Read the model definition and answer for the solid it produces. Units are mm, in the model's axes. A direction names the side the tool comes from. Coordinates: 2 decimals unless noted, no trailing zeros. Write each loop counter-clockwise with the first axis right and the second up, starting at its lowest first coordinate (ties: lowest second). Pieces come first, ordered by that corner, then holes. Notation, with made-up numbers: (0, -24) - (59, -24) arc R33 cw to (59, 11) - close; hole circle Ø2 at (-25.5, -36.5). An arc over 180 degrees is marked (long way). Return JSON: item names as keys, results as strings.
```python
from build123d import *
from OCP.BRepFilletAPI import BRepFilletAPI_MakeChamfer

# Parameters (mm, degrees)
SKETCH1_R           = 4
SKETCH1_R_2         = 1.6
BOSS_EXTRUDE1_DEPTH = 23
SKETCH3_W           = 13.555932204
SKETCH3_H           = 6
SKETCH3_R           = 1.6
CUT_EXTRUDE1_DEPTH  = 2
BOSS_EXTRUDE2_DEPTH = 4
CHAMFER1_SIZE       = 1.5
CHAMFER1_SIZE_2     = 1.062746067


with BuildPart() as part:
    # Sketch1 → Boss-Extrude1 (new body)
    with BuildSketch(Plane(origin=(0, 0, 0), x_dir=(1, 0, 0), z_dir=(0, 1, 0))):
        with Locations(Location((0, 0, 0), (0, 0, 270))):
            Circle(SKETCH1_R)
        with Locations(Location((0, 0, 0), (0, 0, 270))):
            Circle(SKETCH1_R_2, mode=Mode.SUBTRACT)
    extrude(amount=BOSS_EXTRUDE1_DEPTH)

    # Sketch3 → Cut-Extrude1 (cut)
    with BuildSketch(Plane.XZ):
        Rectangle(SKETCH3_W, SKETCH3_H)
        with Locations(Location((0, 0, 0), (0, 0, 270))):
            Circle(SKETCH3_R, mode=Mode.SUBTRACT)
    extrude(amount=-CUT_EXTRUDE1_DEPTH, mode=Mode.SUBTRACT)

    # Sketch5 → Boss-Extrude2 (add)
    with BuildSketch(Plane.XZ):
        with BuildLine():
            Line((-4.609772229, 3), (4.609772229, 3))
            ThreePointArc((4.609772229, 3), (0, 5.5), (-4.609772229, 3))
        make_face()
        with BuildLine():
            Line((4.609772229, -3), (-4.609772229, -3))
            ThreePointArc((-4.609772229, -3), (0, -5.5), (4.609772229, -3))
        make_face()
    extrude(amount=-BOSS_EXTRUDE2_DEPTH)

    # Chamfer1
    chamfer1_edges_1 = [part.edges().sort_by_distance(p)[0] for p in [
        (2.645751311, 3, -3),
    ]]
    chamfer1_side_1 = [part.faces().sort_by_distance(p)[0] for p in [
        (2.667006232, 3, -3),
    ]]
    chamfer1_edges_2 = [part.edges().sort_by_distance(p)[0] for p in [
        (-2.645751311, 3, -3),
    ]]
    chamfer1_side_2 = [part.faces().sort_by_distance(p)[0] for p in [
        (-2.667006232, 3, -3),
    ]]
    chamfer1_edges_3 = [part.edges().sort_by_distance(p)[0] for p in [
        (2.645751311, 3, 3),
    ]]
    chamfer1_side_3 = [part.faces().sort_by_distance(p)[0] for p in [
        (2.667006232, 3, 3),
    ]]
    chamfer1_edges_4 = [part.edges().sort_by_distance(p)[0] for p in [
        (-2.645751311, 3, 3),
    ]]
    chamfer1_side_4 = [part.faces().sort_by_distance(p)[0] for p in [
        (-2.667006232, 3, 3),
    ]]
    chamfer1_edges_5 = [part.edges().sort_by_distance(p)[0] for p in [
        (1.414213562, 4, 3.741657387),
        (0, 4, -4),
    ]]
    chamfer1 = BRepFilletAPI_MakeChamfer(part.part.solid().wrapped)
    for e in chamfer1_edges_1:
        chamfer1.Add(CHAMFER1_SIZE - 0.0001, CHAMFER1_SIZE_2 - 0.0001, e.wrapped, chamfer1_side_1[0].wrapped)
    for e in chamfer1_edges_2:
        chamfer1.Add(CHAMFER1_SIZE - 0.0001, CHAMFER1_SIZE_2 - 0.0001, e.wrapped, chamfer1_side_2[0].wrapped)
    for e in chamfer1_edges_3:
        chamfer1.Add(CHAMFER1_SIZE - 0.0001, CHAMFER1_SIZE_2 - 0.0001, e.wrapped, chamfer1_side_3[0].wrapped)
    for e in chamfer1_edges_4:
        chamfer1.Add(CHAMFER1_SIZE - 0.0001, CHAMFER1_SIZE_2 - 0.0001, e.wrapped, chamfer1_side_4[0].wrapped)
    for e in chamfer1_edges_5:
        chamfer1.Add(CHAMFER1_SIZE - 0.0001, e.wrapped)
    add(Compound.cast(chamfer1.Shape()), mode=Mode.REPLACE)  # a hair under: the kernel refuses the full size


solid = part.part
```
(1) A cutting plane is placed at A-A (y = 3). Determine the outline of the cut face in (x, z), and give its area (3 significant figures).
Answer:
{"outline": "(-4.61, -3) arc R5.5 ccw to (4.61, -3) - (4.15, -3) - (3.34, -2.2) arc R4 ccw to (3.34, 2.2) - (4.15, 3) - (4.61, 3) arc R5.5 ccw to (-4.61, 3) - (-4.15, 3) - (-3.34, 2.2) arc R4 ccw to (-3.34, -2.2) - (-4.15, -3) - close; hole circle Ø3.2 at (0, 0)", "area": "69.7 mm²"}
(2) Flat-ended cylindrical pins translate along their axes: P1, Ø4, axis at y = 10, z = -3.5, coming from the +X side; P2, Ø6, axis at y = 16.5, z = -2, coming from the -X side; P3, Ø1.5, axis at y = 2.5, z = 0.5, coming from the +X side. Find the tip coordinate at first contact, or state that the pin passes through.
Answer:
{"P1": "x = 3.71", "P2": "x = -4", "P3": "x = 4"}
(3) Straight lines are drawn through the part: line 1 (X direction, y = 6.75, z = 0); line 2 (Y direction, x = 2.25, z = 1.5); line 3 (X direction, y = 3.75, z = -1.25). For each, find the intervals that lie inside material, in ascending order. Write a range as from..to.
Answer:
{"line 1": "-4..-1.6, 1.6..4", "line 2": "2..23", "line 3": "-3.8..-1, 1..3.8"}
(4) Determine the mould class of faces 1 (the face through (-2, 2, 0)), 2 (the face through (0, 0, -4)), 3 (the face through (0.1, 5.1, 4.4)) for opening direction Z: +Z half, -Z half, draft (parallel to the pull), parting line (faces both ways), or undercut.
Answer:
{"face 1": "undercut", "face 2": "draft", "face 3": "+Z half"}
(5) A cutting plane is placed at B-B (z = 0). Determine the outline of the cut face in (x, y), and give its area (3 significant figures).
Answer:
{"outline": "(-4, 2) - (-1.6, 2) - (-1.6, 23) - (-4, 23) - close; (1.6, 2) - (4, 2) - (4, 23) - (1.6, 23) - close", "area": "101 mm²"}
(6) A cutting plane is placed at C-C (y = 5.75). Determine the outline of the cut face in (x, z), and give its area (3 significant figures).
Answer:
{"outline": "circle Ø8 at (0, 0); hole circle Ø3.2 at (0, 0)", "area": "42.2 mm²"}
(7) Which of the six approach directions +Z, -Z, +X, -X, +Y, -Y give full straight-line access (tool end or side, diameter ignored) to faces 4 (the face through (3.738, 3.386, -2.593)), 5 (the face through (-1.532, 12.353, 3.695)), 6 (the face through (-3.738, 3.386, 2.593))?
Answer:
{"face 4": "+X, +Y, -Y", "face 5": "+Y", "face 6": "-X, +Y, -Y"}
